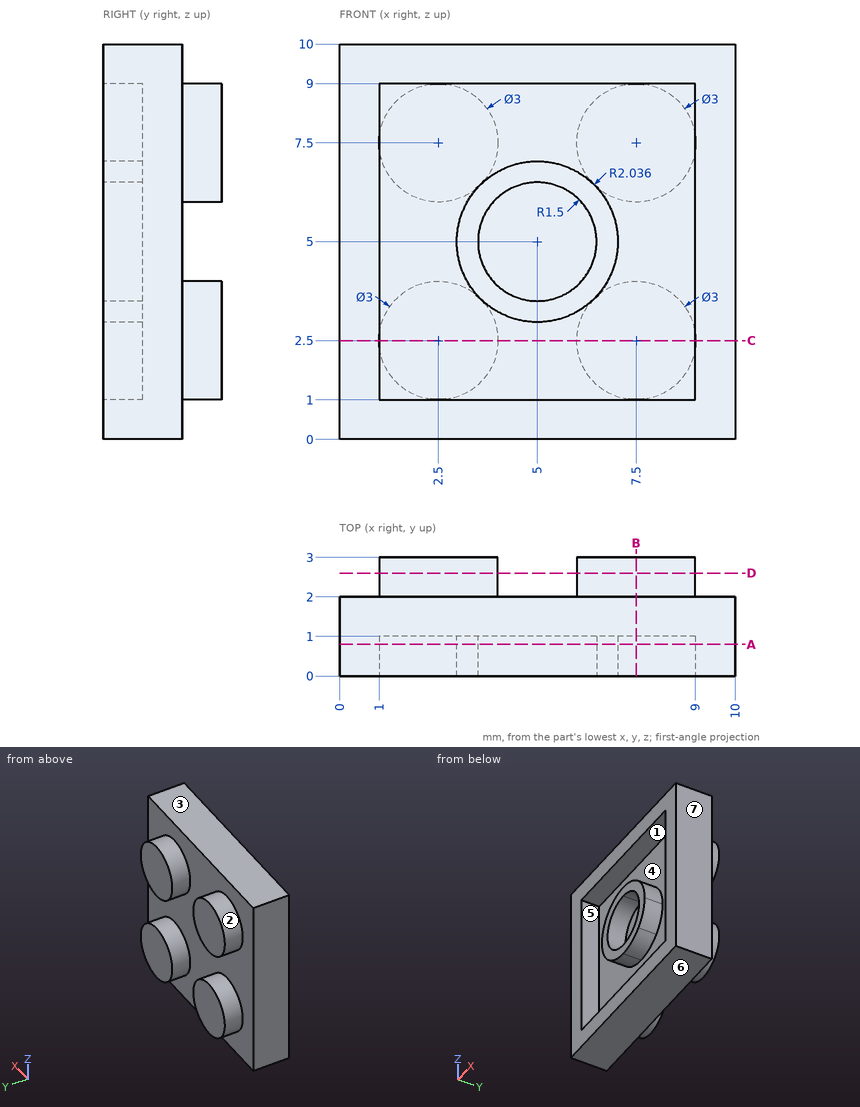
For this review, use the dimensioned drawing (mm, ordinates from the lowest corner) and the shaded views. A direction names the side the tool comes from. Give positions to 0.01 mm unless a question says otherwise; leave off trailing zeros. Order: outer loops, then holes, each group sorted by start corner. A loop starts at its lowest first (then second) coordinate and runs counter-clockwise, first axis right, second up.
1) Wall thickness on line 1 (X direction, y = 0.65, z = 5.25); line 2 (Z direction, x = 6, y = 0.2) (1 decimal); line 3 (X direction, y = 0.2, z = 6.25) (1 decimal): over which ranges is each line inside the solid? List them lowest first.
2) Insertion check: pin 1 (0.9 mm diameter, centred on x = 5.5, z = 4.5, fed in from -Y); pin 2 (2 mm diameter, centred on x = 5.5, z = 5.5, fed in from +Y). Each pin has a flat end and moves straight along its axis. Give the tip position at first contact, or say it passes through.
3) Take a section at B-B (x = 7.5). Give the boundary of the cut face in (y, z), then the cut area to 3 significant figures.
4) Take a section at D-D (y = 2.6). Give the boundary of the cut face in (x, z).
5) Take a section at C-C (z = 2.5). Give the boundary of the cut face in (x, y), then the cut area to 3 significant figures.
6) Take a section at A-A (y = 0.8). Give the boundary of the cut face in (x, z) (1 decimal).
7) For the marked faces 1, 2 and 3, list the 3-axis set-ups (+Z, -Z, +X, -X, +Y, -Y) from which the entire face can be reached by the end or side of a thin tool; tool diameter is ignored.
8) The part is to be moulded in two halves that separate along Z. For the marked faces 4, 5, 6 and 7, say which applies: released by +Z, released by -Z, zero draft, split by the parting line, or undercut.
Derived:
1. line 1: x = 0 to 1, 2.98 to 3.52, 6.48 to 7.02, 9 to 10
1. line 2: z = 0 to 1, 3.2 to 3.9, 6.1 to 6.8, 9 to 10
1. line 3: x = 0 to 1, 3.4 to 4.2, 5.8 to 6.6, 9 to 10
2. pin 1: stops at y = 1
2. pin 2: stops at y = 2
3. outline: (0, 0) - (2, 0) - (2, 1) - (3, 1) - (3, 4) - (2, 4) - (2, 6) - (3, 6) - (3, 9) - (2, 9) - (2, 10) - (0, 10) - (0, 9) - (1, 9) - (1, 1) - (0, 1) - close
3. area: 18.0 mm2
4. outline: circle Ø3 at (2.5, 2.5); circle Ø3 at (2.5, 7.5); circle Ø3 at (7.5, 2.5); circle Ø3 at (7.5, 7.5)
5. outline: (0, 0) - (1, 0) - (1, 1) - (9, 1) - (9, 0) - (10, 0) - (10, 2) - (9, 2) - (9, 3) - (6, 3) - (6, 2) - (4, 2) - (4, 3) - (1, 3) - (1, 2) - (0, 2) - close
5. area: 18.0 mm2
6. outline: (0, 0) - (10, 0) - (10, 10) - (0, 10) - close; circle Ø4.1 at (5, 5); hole (1, 1) - (9, 1) - (9, 9) - (1, 9) - close; hole circle Ø3 at (5, 5)
7. face 1: -Y
7. face 2: +Y
7. face 3: +Z, +X, -X, +Y, -Y
8. face 4: undercut
8. face 5: undercut
8. face 6: released by -Z
8. face 7: zero draft
